For this review, use the dimensioned drawing (mm, ordinates from the lowest corner) and the shaded views. A direction names the side the tool comes from. Round coordinates to 2 decimals unless told otherwise and drop trailing zeros. Loops run counter-clockwise (first coordinate to the right, second up) from the corner with the lowest first, then second, coordinate; pieces in that order, holes last. Notation, with made-up numbers: (51.5, 41.5) - (71.5, 41.5) arc R26 ccw to (71.5, 71.5) - close; hole circle Ø8 at (3, 6). An arc over 180 degrees is marked (long way). Use one line per item in the form item = value. Start each with the question number.
(1) The part is to be moulded in two halves that separate along Z. For the marked faces 1, 2 and 3, say which applies: released by +Z, released by -Z, zero draft, split by the parting line, or undercut.
(2) For pin 1 (5 mm diameter, centred on x = 6.42, z = 10.73, fed in from -Y); pin 2 (6 mm diameter, centred on x = 12, y = 10, fed in from -Z); pin 3 (1.5 mm diameter, centred on x = 8, y = 12, fed in from -Z), all flat-tipped, find the tip position at first contact; note any pin that passes through.
(3) Wall thickness on probe 1 along Z at (x, y) = (16.6, 9.25); probe 2 along Y at (x, z) = (6, 25); probe 3 along X at (y, z) = (2.5, 14.5): over which ranges is each line inside the solid? List them lowest first. Write a range as [from, to].
(4) We need section A-A, the plane x = 16.6. Write out the cut boundary in (y, z), then the cut area to 3 significant figures.
(5) We need section D-D, the plane x = 7. Write out the cut boundary in (y, z), then the cut area to 3 significant figures.
(6) We need section B-B, the plane z = 16.6. Write out the cut boundary in (x, y).
(7) Machinability: for the marked faces 4 and 5, which of the approach directions +Z, -Z, +X, -X, +Y, -Y give a long, thin tool a straight path to every point of the face, cutting with its end or side? Answer none if there is none.
(8) We need section C-C, the plane y = 3.25. Write out the cut boundary in (x, z), then the cut area to 3 significant figures.
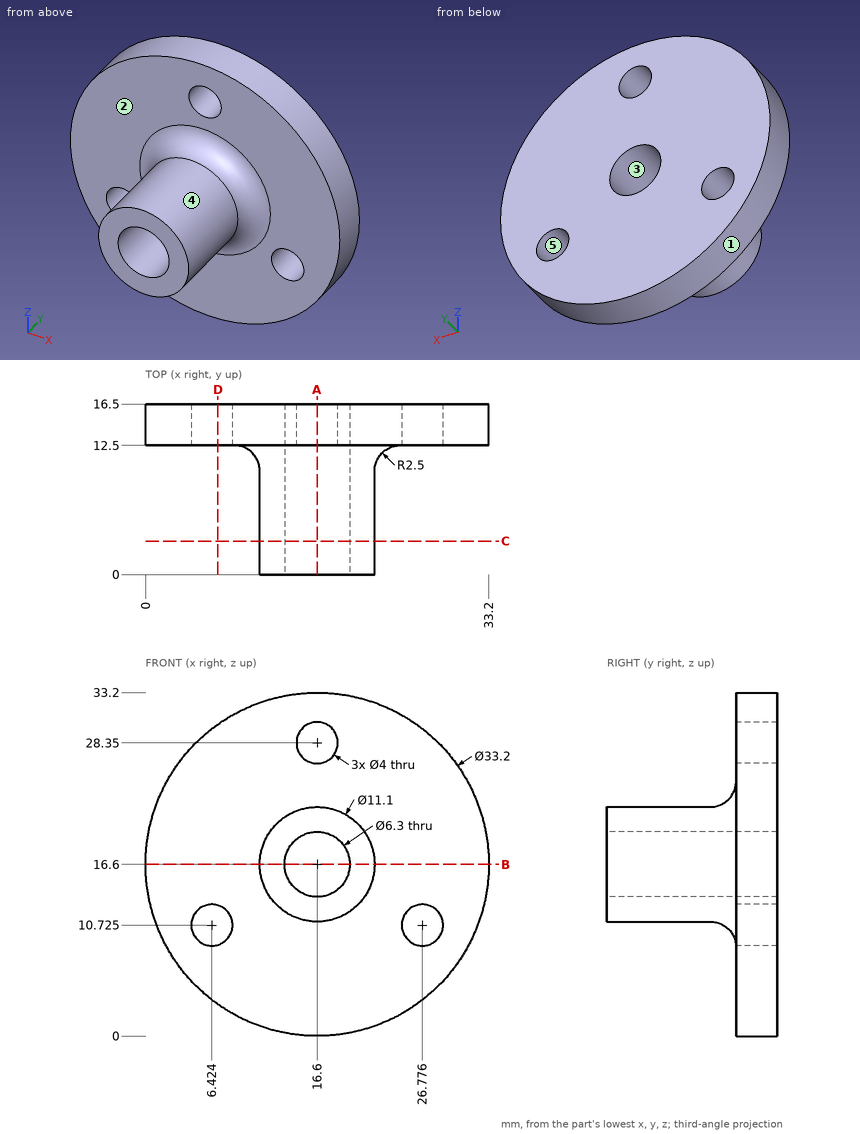
Data:
q1.face_1 = split by the parting line
q1.face_2 = zero draft
q1.face_3 = undercut
q2.pin_1 = 12.5
q2.pin_2 = 0.26
q2.pin_3 = 2.08
q3.probe_1 = [11.05, 13.45], [19.75, 22.15]
q3.probe_2 = [12.5, 16.5]
q3.probe_3 = [11.46, 14.25], [18.95, 21.74]
q4.outline = (0, 11.05) - (10, 11.05) arc R2.5 cw to (12.5, 8.55) - (12.5, 0) - (16.5, 0) - (16.5, 13.45) - (0, 13.45) - close; (0, 19.75) - (16.5, 19.75) - (16.5, 26.35) - (12.5, 26.35) - (12.5, 24.65) arc R2.5 cw to (10, 22.15) - (0, 22.15) - close; (12.5, 30.35) - (16.5, 30.35) - (16.5, 33.2) - (12.5, 33.2) - close
q4.area = 154 mm^2
q5.outline = (12.5, 3.06) - (16.5, 3.06) - (16.5, 8.81) - (12.5, 8.81) - close; (12.5, 12.64) - (16.5, 12.64) - (16.5, 30.14) - (12.5, 30.14) - close
q5.area = 93.0 mm^2
q6.outline = (0, 12.5) - (8.55, 12.5) arc R2.5 cw to (11.05, 10) - (11.05, 0) - (13.45, 0) - (13.45, 16.5) - (0, 16.5) - close; (19.75, 0) - (22.15, 0) - (22.15, 10) arc R2.5 cw to (24.65, 12.5) - (33.2, 12.5) - (33.2, 16.5) - (19.75, 16.5) - close
q7.face_4 = -Y
q7.face_5 = +Y, -Y
q8.outline = circle Ø11.1 at (16.6, 16.6); hole circle Ø6.3 at (16.6, 16.6)
q8.area = 65.6 mm^2
